Here's how the part is built. I have some questions about the finished solid (model axes, mm). A direction names the side the tool comes from. Give positions to 0.01 mm unless a question says otherwise; leave off trailing zeros. Loops run counter-clockwise (first coordinate to the right, second up) from the corner with the lowest first, then second, coordinate; pieces in that order, holes last.
Q1. I'm going to push flat-ended pins straight in: P1, Ø0.7, axis at y = -1.5, z = 0.5, coming from the +X side; P2, Ø1, axis at x = 5, z = 1.5, coming from the +Y side; P3, Ø0.5, axis at x = -3.5, y = 3.5, coming from the +Z side (3 decimals); P4, Ø4, axis at x = 4.5, y = -0.5, coming from the +Z side (3 decimals). Where does each tip first touch, or does it pass through?
Q2. Suppose I cut it at A-A (y = 1). List the corners of the cut face in (x, z) for me (3 decimals), and give its area (3 significant figures).
Q3. Thinking about a two-plate mould opening in Z: for faces 4 (the face through (0, 0, 0)), 5 (the face through (0, 3, 2.875)), 6 (the face through (-5.4, 4, 0)), 7 (the face through (0, 3, -2.875)), which applies, pulls with the +Z half, pulls with the -Z half, needs draft (parallel to the pull), parting line crosses it, or undercut?
Q4. Suppose I cut it at B-B (z = 1.15). List the corners of the cut face in (x, y) for me.
Q5. I need wall thicknesses on probe 1 along Z at (x, y) = (1.5, 2.25) (3 decimals); probe 2 along X at (y, z) = (6, -1.1); probe 3 along Z at (x, y) = (2, 5.75) (3 decimals). Which ranges of each line are inside material? Lowest first, please.
Q6. For faces 1 (the face through (5.4, 4, 0)), 2 (the face through (-5.9, 3.8, 1.5)), 3 (the face through (6.2, 3, 0)), which set-ups out of +Z, -Z, +X, -X, +Y, -Y let a thin tool reach every point of the face, with its end or its side?
Q7. Suppose I cut it at C-C (x = 2.75). List the corners of the cut face in (y, z) for me (3 decimals).
Q8. Suppose I cut it at D-D (y = 4.75). Count the separate pieces of the cut face and the enclosed holes in it, and give its area (3 significant figures).
```python
from build123d import *

# Parameters (mm, degrees)
SKETCH1_W                = 12.4
SKETCH1_H                = 5.75
BOSS_EXTRUDE1_DEPTH      = 7
SHELL1_T                 = -0.8
SKETCH2_W                = 1.25
SKETCH2_H                = 3.2
CUT_EXTRUDE1_DEPTH       = 13.4
CUT_EXTRUDE2_REACH       = 7.75
SKETCH3_W                = 1.7
SKETCH3_H                = 3.8
SKETCH4_W                = 0.64
SKETCH4_H                = 0.64
BOSS_EXTRUDE2_DEPTH      = 3.45
BOSS_EXTRUDE2_DEPTH_BACK = 6.75
CHAMFER1_SIZE            = 0.2


with BuildPart() as part:
    # Sketch1 → Boss-Extrude1 (new body)
    with BuildSketch(Plane(origin=(0, 0, 0), x_dir=(1, 0, 0), z_dir=(0, 1, 0))):
        Rectangle(SKETCH1_W, SKETCH1_H)
    extrude(amount=BOSS_EXTRUDE1_DEPTH)

    # Shell1
    shell1_openings = [part.faces().sort_by_distance(p)[0] for p in [
        (0, 7, 0),
    ]]
    offset(amount=SHELL1_T, openings=shell1_openings, kind=Kind.INTERSECTION)

    # Sketch2 → Cut-Extrude1 (cut, through all)
    with BuildSketch(Plane(origin=(6.2, 0, 0), x_dir=(0, 0, -1), z_dir=(1, 0, 0))):
        with Locations((-1.5, 5.4)):
            Rectangle(SKETCH2_W, SKETCH2_H)
    extrude(amount=-CUT_EXTRUDE1_DEPTH, mode=Mode.SUBTRACT)

    # Sketch3 → Cut-Extrude2 (cut, up to next)
    with BuildSketch(Plane.XY.offset(2.875), mode=Mode.PRIVATE) as cut_extrude2_sk1:
        with Locations((-3.45, 5.1)):
            Rectangle(SKETCH3_W, SKETCH3_H)
    cut_extrude2_tool1 = extrude(cut_extrude2_sk1.sketch, amount=-CUT_EXTRUDE2_REACH, mode=Mode.PRIVATE) & part.part
    add(cut_extrude2_tool1.solids().sort_by_distance((-3.45, 5.1, 2.875))[0], mode=Mode.SUBTRACT)
    # Sketch3 → Cut-Extrude2 (cut, up to next)
    with BuildSketch(Plane.XY.offset(2.875), mode=Mode.PRIVATE) as cut_extrude2_sk2:
        with Locations((3.45, 5.1)):
            Rectangle(SKETCH3_W, SKETCH3_H)
    cut_extrude2_tool2 = extrude(cut_extrude2_sk2.sketch, amount=-CUT_EXTRUDE2_REACH, mode=Mode.PRIVATE) & part.part
    add(cut_extrude2_tool2.solids().sort_by_distance((3.45, 5.1, 2.875))[0], mode=Mode.SUBTRACT)

    # Sketch4 → Boss-Extrude2 (add, two sides)
    with BuildSketch(Plane.XZ) as boss_extrude2_sk:
        with Locations((-3.75, 0.525)):
            Rectangle(SKETCH4_W, SKETCH4_H)
        with Locations((-1.21, 0.525)):
            Rectangle(SKETCH4_W, SKETCH4_H)
        with Locations((1.33, 0.525)):
            Rectangle(SKETCH4_W, SKETCH4_H)
        with Locations((3.87, 0.525)):
            Rectangle(SKETCH4_W, SKETCH4_H)
    extrude(amount=BOSS_EXTRUDE2_DEPTH)
    extrude(boss_extrude2_sk.sketch, amount=-BOSS_EXTRUDE2_DEPTH_BACK)

    # Chamfer1
    chamfer1_edges = [part.edges().sort_by_distance(p)[0] for p in [
        (-1.21, 6.75, 0.205),
        (-1.53, 6.75, 0.525),
        (-1.21, 6.75, 0.845),
        (-0.89, 6.75, 0.525),
        (-1.21, -3.45, 0.205),
        (-0.89, -3.45, 0.525),
        (-1.21, -3.45, 0.845),
        (-1.53, -3.45, 0.525),
        (1.33, 6.75, 0.205),
        (1.01, 6.75, 0.525),
        (1.33, 6.75, 0.845),
        (1.65, 6.75, 0.525),
        (1.33, -3.45, 0.205),
        (1.65, -3.45, 0.525),
        (1.33, -3.45, 0.845),
        (1.01, -3.45, 0.525),
        (3.87, 6.75, 0.205),
        (3.55, 6.75, 0.525),
        (3.87, 6.75, 0.845),
        (4.19, 6.75, 0.525),
        (3.87, -3.45, 0.205),
        (4.19, -3.45, 0.525),
        (3.87, -3.45, 0.845),
        (3.55, -3.45, 0.525),
        (-3.43, 6.75, 0.525),
        (-3.75, 6.75, 0.205),
        (-4.07, 6.75, 0.525),
        (-3.75, 6.75, 0.845),
        (-3.43, -3.45, 0.525),
        (-3.75, -3.45, 0.845),
        (-4.07, -3.45, 0.525),
        (-3.75, -3.45, 0.205),
    ]]
    chamfer(chamfer1_edges, length=CHAMFER1_SIZE)


solid = part.part
```
Solutions:
1. P1: stops at x = 4.19
1. P2: stops at y = 3.8
1. P3: stops at z = 0.845
1. P4: stops at z = 2.875
2. outline: (-6.2, -2.875) - (6.2, -2.875) - (6.2, 2.875) - (-6.2, 2.875) - close; (-4.07, 0.205) - (-3.43, 0.205) - (-3.43, 0.845) - (-4.07, 0.845) - close; (-1.53, 0.205) - (-0.89, 0.205) - (-0.89, 0.845) - (-1.53, 0.845) - close; (1.01, 0.205) - (1.65, 0.205) - (1.65, 0.845) - (1.01, 0.845) - close; (3.55, 0.205) - (4.19, 0.205) - (4.19, 0.845) - (3.55, 0.845) - close; hole (-5.4, -2.075) - (5.4, -2.075) - (5.4, 2.075) - (-5.4, 2.075) - close
2. area: 28.1 mm2
3. face 4: needs draft
3. face 5: pulls with the +Z half
3. face 6: undercut
3. face 7: pulls with the -Z half
4. outline: (-6.2, 0) - (6.2, 0) - (6.2, 3.8) - (5.4, 3.8) - (5.4, 0.8) - (-5.4, 0.8) - (-5.4, 3.8) - (-6.2, 3.8) - close
5. probe 1: z = -2.875 to -2.075, 0.205 to 0.845, 2.075 to 2.875
5. probe 2: x = -6.2 to -5.4, 5.4 to 6.2
5. probe 3: z = -2.875 to -2.075, 2.125 to 2.875
6. face 1: +Y
6. face 2: +X, -X, +Y
6. face 3: +Z, -Z, +X, +Y, -Y
7. outline: (0, -2.875) - (7, -2.875) - (7, -2.075) - (0.8, -2.075) - (0.8, 2.075) - (3.2, 2.075) - (3.2, 2.875) - (0, 2.875) - close
8. separate pieces: 8
8. enclosed holes: 0
8. area: 23.0 mm2
